Can you work these out from the model? Positions are in its coordinate system, mm. Face numbers are marked on the shaded views. A direction names the side the tool comes from. Coordinates: 2 decimals unless noted, no trailing zeros. Order: outer loops, then holes, each group sorted by start corner. A loop starts at its lowest first (then second) coordinate and runs counter-clockwise, first axis right, second up. Notation, with made-up numbers: (82, 13) - (107, 13) arc R27 ccw to (107, 46) - close; hole circle Ø6 at (-18, -30). An arc over 180 degrees is marked (long way). Use a Markdown table: item, result. Add a question column.
(1) I want a section at B-B (z = 0.7). State how many separate pieces and enclosed holes the cut face has, and give its area (3 significant figures).
(2) We'd pull the mould along Y, two halves only. Please class the marked faces 1, 2 and 3: pulls with the +Y half, pulls with the -Y half, needs draft (parallel to the pull), parting line crosses it, or undercut.
(3) I want a section at A-A (x = -12.7). List the corners of the cut face in (y, z) for me (1 decimal), and give its area (3 significant figures).
(4) On a 3-axis mill with a long thin cutter (end or side, diameter ignored), from which of +Z, -Z, +X, -X, +Y, -Y can I reach the whole of each face in a straight line? I mean the marked faces 4 and 5. Say none if no direction works.
(5) For pin 1 Ø1.5 at (x, z) = (-41.5, 1.5) entering from +Y; pin 2 Ø1.5 at (x, z) = (-30, 0.5) entering from -Y; pin 3 Ø5 at (x, y) = (-12.7, 4.445) entering from -Z; pin 4 Ø1.9 at (x, y) = (-12.7, -4.445) entering from -Z, each with a flat end and sliding along its axis, tell me the tip position at first contact or that it passes through.
(6) I want a section at D-D (y = -14.5). List the corners of the cut face in (x, z) for me (3 decimals).
(7) I want a section at C-C (x = -48). List the corners of the cut face in (y, z) for me (1 decimal).
(8) If I drill on L1, parallel to Y at x = -12.7, z = 0.7; L2, parallel to Y at x = -32.5, z = 1.65; L3, parallel to Y at x = -30, z = 0.6, over which ranges is the centre line in solid material (lowest first)? Write a range as [from, to].
```python
from build123d import *

# Parameters (mm, degrees)
F0_R     = 1.5875
F1_DEPTH = 3.175
F2_R     = 5.08
F3_R     = 5.08
F4_R     = 2.54
F5_R     = 5.08


with BuildPart() as f1:
    # F0 (on Top) → F1 (new body)
    with BuildSketch(Plane.XY):
        with BuildLine():
            ThreePointArc((-50.8, 0), (-47.7363851359, -17.3746232809), (-38.9150577104, -32.6536105721))
            Line((-38.9150577104, -32.6536105721), (-29.1862932828, -24.4902079291))
            ThreePointArc((-29.1862932828, -24.4902079291), (-34.023485561, -17.14679067), (-37.0483184504, -8.89))
            Line((-37.0483184504, -8.89), (-6.35, -8.89))
            Line((-6.35, -8.89), (-6.35, 0))
            Line((-6.35, 0), (-6.35, 8.89))
            Line((-6.35, 8.89), (-37.0483184504, 8.89))
            ThreePointArc((-37.0483184504, 8.89), (-34.023485561, 17.14679067), (-29.1862932828, 24.4902079291))
            Line((-29.1862932828, 24.4902079291), (-38.9150577104, 32.6536105721))
            ThreePointArc((-38.9150577104, 32.6536105721), (-47.7363851359, 17.3746232809), (-50.8, 0))
        make_face()
        with Locations((-12.7, -4.445)):
            Circle(F0_R, mode=Mode.SUBTRACT)
        with Locations((-12.7, 4.445)):
            Circle(F0_R, mode=Mode.SUBTRACT)
    extrude(amount=F1_DEPTH)

    # F2
    f2_edges = [f1.edges().sort_by_distance(p)[0] for p in [
        (-38.915058, 32.653611, 1.5875),
        (-38.915058, -32.653611, 1.5875),
    ]]
    fillet(f2_edges, radius=F2_R)

    # F3
    f3_edges = [f1.edges().sort_by_distance(p)[0] for p in [
        (-29.186293, 24.490208, 1.5875),
        (-29.186293, -24.490208, 1.5875),
    ]]
    fillet(f3_edges, radius=F3_R)

    # F4
    f4_edges = [f1.edges().sort_by_distance(p)[0] for p in [
        (-37.048318, -8.89, 1.5875),
        (-37.048318, 8.89, 1.5875),
    ]]
    fillet(f4_edges, radius=F4_R)

    # F5
    f5_edges = [f1.edges().sort_by_distance(p)[0] for p in [
        (-6.35, 8.89, 1.5875),
        (-6.35, -8.89, 1.5875),
    ]]
    fillet(f5_edges, radius=F5_R)


solid = f1.part
```
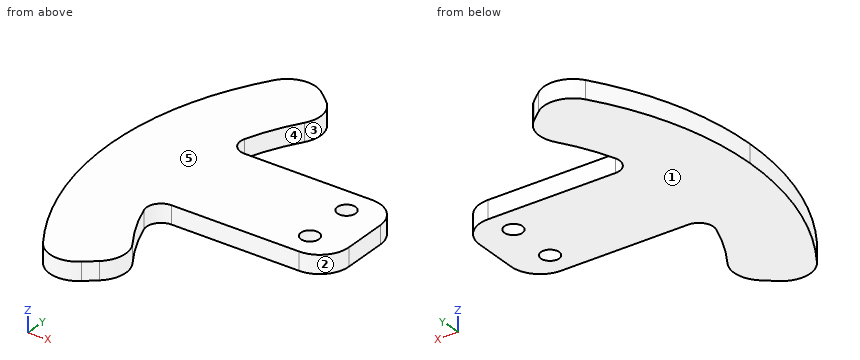
Answers follow:
| question | item | result |
|---|---|---|
| 1 | separate pieces | 1 |
| 1 | enclosed holes | 2 |
| 1 | area | 1,300 mm² |
| 2 | face 1 | needs draft |
| 2 | face 2 | pulls with the -Y half |
| 2 | face 3 | undercut |
| 3 | outline | (-8.9, 0) - (-6, 0) - (-6, 3.2) - (-8.9, 3.2) - close; (-2.9, 0) - (2.9, 0) - (2.9, 3.2) - (-2.9, 3.2) - close; (6, 0) - (8.9, 0) - (8.9, 3.2) - (6, 3.2) - close |
| 3 | area | 36.3 mm² |
| 4 | face 4 | +Z, -Z, +X |
| 4 | face 5 | +Z, +X, -X, +Y, -Y |
| 5 | pin 1 | stops at y = 29.63 |
| 5 | pin 2 | stops at y = -8.89 |
| 5 | pin 3 | stops at z = 0 |
| 5 | pin 4 | passes through |
| 6 | outline | (-48.687, 0) - (-35.233, 0) - (-35.233, 3.175) - (-48.687, 3.175) - close |
| 7 | outline | (-16.6, 0) - (16.6, 0) - (16.6, 3.2) - (-16.6, 3.2) - close |
| 8 | L1 | y = [-8.89, -6.03], [-2.86, 2.86], [6.03, 8.89] |
| 8 | L2 | y = [-27.24, -19.88], [-8.89, 8.89], [19.88, 27.24] |
| 8 | L3 | y = [-8.89, 8.89] |
